from build123d import *

# Parameters (mm, degrees)
SKETCH1_R           = 3.5
SKETCH1_R_2         = 1.5
BOSS_EXTRUDE1_DEPTH = 11.5
BOSS_EXTRUDE2_DEPTH = 11.5
BOSS_EXTRUDE3_DEPTH = 34.5


with BuildPart() as part:
    # Sketch1 → Boss-Extrude1 (new, symmetric)
    with BuildSketch(Plane.XY):
        Circle(SKETCH1_R)
        Circle(SKETCH1_R_2, mode=Mode.SUBTRACT)
    extrude(amount=BOSS_EXTRUDE1_DEPTH, both=True)

    # Sketch2 → Boss-Extrude2 (add, symmetric)
    with BuildSketch(Plane.XY):
        with BuildLine():
            Line((0, -3.5), (-15, -3.5))
            Line((-15, -3.5), (-1.548998946, 3.138566913))
            ThreePointArc((-1.548998946, 3.138566913), (-3.408444234, -0.795303655), (0, -3.5))
        make_face()
    extrude(amount=BOSS_EXTRUDE2_DEPTH, both=True)

    # Sketch3 → Boss-Extrude3 (add, symmetric)
    with BuildSketch(Plane(origin=(0, 0, 0), x_dir=(-1, 0, 0), z_dir=(0, 0, -1))):
        with BuildLine():
            Line((3.570714214, -3.5), (15, -3.5))
            Line((15, -3.5), (4.081424237, 1.888721293))
            ThreePointArc((4.081424237, 1.888721293), (4.618328991, -0.880724885), (3.570714214, -3.5))
        make_face()
    extrude(amount=BOSS_EXTRUDE3_DEPTH, both=True)


solid = part.part
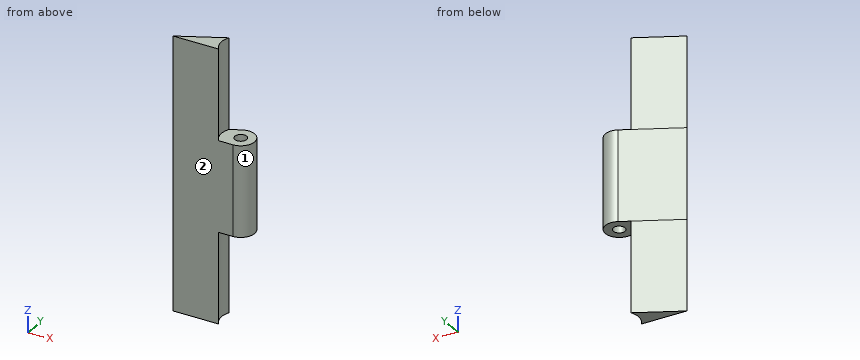
Model file for the job. Use its own axes, mm. Face numbers are marked on the shaded views. Give positions to 0.01 mm unless a question says otherwise; leave off trailing zeros. Write each loop counter-clockwise with the first axis right and the second up, starting at its lowest first coordinate (ties: lowest second). Pieces come first, ordered by that corner, then holes. Notation, with made-up numbers: (10.25, 14.5) -> (18.25, 14.5) arc R22 ccw to (18.25, 28.5) -> close; hole circle Ø2 at (57.5, 30). An arc over 180 degrees is marked (long way). Write item = value, one per line.
(1) Mould opens along X. For the marked faces 1 and 2 say: released by +X, released by -X, zero draft, split by the parting line, or undercut.
Determined:
face_1 = split by the parting line
face_2 = zero draft
(2) Slice it at A-A, the plane y = 0. Give the cut face in (x, z).
Determined:
outline = (-7.91, -34.5) -> (-4.62, -34.5) -> (-4.62, -11.5) -> (-1.5, -11.5) -> (-1.5, 11.5) -> (-4.62, 11.5) -> (-4.62, 34.5) -> (-7.91, 34.5) -> close; (1.5, -11.5) -> (3.5, -11.5) -> (3.5, 11.5) -> (1.5, 11.5) -> close
(3) Slice it at B-B, the plane z = -5.5. Give the cut face in (x, y), then the cut area to 3 significant figures.
Determined:
outline = (-15, -3.5) -> (0, -3.5) arc R3.5 ccw (long way) to (-1.55, 3.14) -> close; hole circle Ø3 at (0, 0)
area = 67.5 mm2
(4) Flat gauge pins, fed straight in: P1, Ø1.8, axis at x = 0, y = 0, coming from the -Z side; P2, Ø2, axis at x = -6.5, z = -0.5, coming from the +Y side; P3, Ø1.5, axis at x = -3.5, z = 4, coming from the +Y side; P4, Ø2, axis at x = 1.5, y = 2.5, coming from the +Z side. Where does each tip first touch, or does it go through?
Determined:
P1 = through
P2 = 1.19
P3 = 2.55
P4 = 11.5
(5) Slice it at D-D, the plane x = -7.5. Give the cut face in (y, z).
Determined:
outline = (-3.5, -34.5) -> (0.2, -34.5) -> (0.2, 34.5) -> (-3.5, 34.5) -> close
(6) Probe line 1 along Y through (x, z) = (0, -4); line 2 along Z through (x, y) = (2.25, 1.25); line 3 along X through (y, z) = (3, 7.5). List the from-to ranges inside material, lowest first.
Determined:
line_1 = -3.5 to -1.5, 1.5 to 3.5
line_2 = -11.5 to 11.5
line_3 = -1.83 to 1.8
(7) Slice it at C-C, the plane z = -16.5. Give the cut face in (x, y).
Determined:
outline = (-15, -3.5) -> (-3.57, -3.5) arc R5 cw to (-4.08, 1.89) -> close
